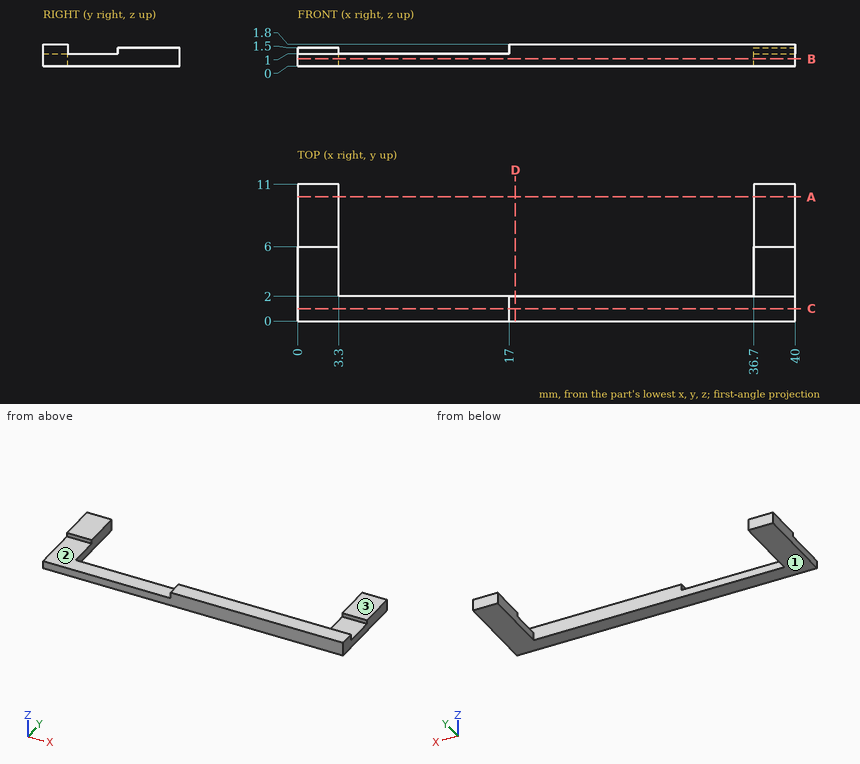
Check sheet for the drawn part. Datum: minimum x, y, z corner. Units: mm. A direction names the side the tool comes from. Round coordinates to 2 decimals unless told otherwise and drop trailing zeros. Loops run counter-clockwise (first coordinate to the right, second up) from the corner with the lowest first, then second, coordinate; pieces in that order, holes last. Notation, with made-up numbers: M 58.5,-16.5 L 92.5,-16.5 A32 ccw 92.5,11.5 Z; hole C -18.75,74 d10. An arc over 180 degrees is marked long. Write each question's results on one line, items separated by ' | '.
1) Gauge pin test, flat ends, axial feed: P1, Ø1.6, axis at x = 39, y = 4.5, coming from the +Z side; P2, Ø2.5, axis at x = 2.5, y = 9, coming from the +Z side. Record the tip position at first contact, or that the pin passes through.
Checks:
P1: stops at z = 1 | P2: stops at z = 1.5
2) Section check B-B on z = 0.6. Record the boundary of the cut face in (x, y), then the cut area to 3 significant figures.
Checks:
outline: M 0,0 L 40,0 L 40,11 L 36.7,11 L 36.7,2 L 3.3,2 L 3.3,11 L 0,11 Z | area: 139 mm2
3) Section check D-D on x = 17.5. Record the boundary of the cut face in (y, z).
Checks:
outline: M 0,0 L 2,0 L 2,1.8 L 0,1.8 Z
4) Section check A-A on y = 10. Record the boundary of the cut face in (x, z).
Checks:
outline: M 0,0 L 3.3,0 L 3.3,1.5 L 0,1.5 Z; M 36.7,0 L 40,0 L 40,1.5 L 36.7,1.5 Z
5) Section check C-C on y = 1. Record the boundary of the cut face in (x, z), then the cut area to 3 significant figures.
Checks:
outline: M 0,0 L 40,0 L 40,1.8 L 17,1.8 L 17,1 L 0,1 Z | area: 58.4 mm2
6) Access from +Z, -Z, +X, -X, +Y, -Y to the whole of each face (thin tool, end or side, straight path). Record for the marked faces 1, 2 and 3.
Checks:
face 1: -Z, +X, -X, +Y, -Y | face 2: +Z, -X, -Y | face 3: +Z, +X, -X, +Y
7) Scan lines: L1, parallel to X at y = 7.75, z = 1.05; L2, parallel to Y at x = 38.5, z = 1.2; L3, parallel to Y at x = 35.5, z = 0.15. Record each from-to range of solid material in increasing order. Write a range as from..to.
Checks:
L1: x = 0..3.3, 36.7..40 | L2: y = 0..2, 6..11 | L3: y = 0..2
